Geometry check sheet. Reference: the model listing, model coordinates, mm. Face numbers are marked on the shaded views. A direction names the side the tool comes from. Coordinates: 2 decimals unless noted, no trailing zeros. Write each loop counter-clockwise with the first axis right and the second up, starting at its lowest first coordinate (ties: lowest second). Pieces come first, ordered by that corner, then holes. Notation, with made-up numbers: M 18,3.25 L 55,3.25 A13 ccw 55,23.25 Z; hole C -39.5,-13.75 d1. An arc over 180 degrees is marked long. Answer as a JSON object with one key per item and string values. Group by question number.
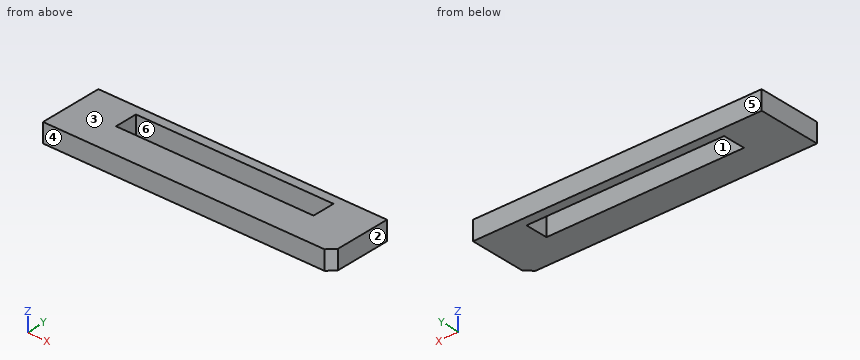
```python
from build123d import *

# Parameters (mm, degrees)
SKETCH_1_W          = 81.1
SKETCH_1_H          = 17.8
EXTRUDE_1_DEPTH     = 5.34
CHAMFER_1_SIZE      = 2
SKETCH_2_W          = 55.5
SKETCH_2_H          = 6.409449073
CUT_EXTRUDE_1_DEPTH = 6.34


with BuildPart() as part:
    # Эскиз1 → Бобышка-Вытянуть1 (new body)
    with BuildSketch(Plane.XY):
        with Locations((40.55, 8.9)):
            Rectangle(SKETCH_1_W, SKETCH_1_H)
    extrude(amount=EXTRUDE_1_DEPTH)

    # Фаска1
    chamfer_1_edges = [part.edges().sort_by_distance(p)[0] for p in [
        (81.1, 0, 2.67),
    ]]
    chamfer(chamfer_1_edges, length=CHAMFER_1_SIZE)

    # Эскиз2 → Вырез-Вытянуть1 (cut, through all)
    with BuildSketch(Plane.XY.offset(5.34)):
        with Locations((40.55, 12.038647742)):
            Rectangle(SKETCH_2_W, SKETCH_2_H)
    extrude(amount=-CUT_EXTRUDE_1_DEPTH, mode=Mode.SUBTRACT)


solid = part.part
```
1) Section check C-C (y = 12). Record the cut outline in (x, z), then the cut area to 3 significant figures.
2) Draft check along Y on the marked faces 3, 4, 5 and 6. Enter one of: +Y half, -Y half, draft (parallel to the pull), parting line (faces both ways), or undercut.
3) Section check A-A (x = 63). Record the cut outline in (y, z), then the cut area to 3 significant figures.
4) Set-up check for the marked faces 1 and 2: record each of +Z, -Z, +X, -X, +Y, -Y from which the full face is reachable in a straight line by a thin tool's end or side.
5) Section check B-B (z = 4). Record the cut outline in (x, y), then the cut area to 3 significant figures.
6) Go/stop test with a flat-tipped pin: pin 1 Ø1.5 at (y, z) = (16, 3.5) entering from -X. Record where the tip stops, or that it passes through.
7) Material ranges on probe 1 along X at (y, z) = (11.75, 4.65); probe 2 along Y at (x, z) = (44, 4.2); probe 3 along X at (y, z) = (1.5, 2.3), recorded low to high. Write a range as [from, to].
Entries:
{
 "1": {"outline": "M 0,0 L 12.8,0 L 12.8,5.34 L 0,5.34 Z; M 68.3,0 L 81.1,0 L 81.1,5.34 L 68.3,5.34 Z", "area": "137 mm^2"},
 "2": {"face 3": "draft", "face 4": "-Y half", "face 5": "+Y half", "face 6": "undercut"},
 "3": {"outline": "M 0,0 L 8.83,0 L 8.83,5.34 L 0,5.34 Z; M 15.24,0 L 17.8,0 L 17.8,5.34 L 15.24,5.34 Z", "area": "60.8 mm^2"},
 "4": {"face 1": "+Z, -Z", "face 2": "+Z, -Z, +X, +Y, -Y"},
 "5": {"outline": "M 0,0 L 79.1,0 L 81.1,2 L 81.1,17.8 L 0,17.8 Z; hole M 12.8,8.83 L 68.3,8.83 L 68.3,15.24 L 12.8,15.24 Z", "area": "1,090 mm^2"},
 "6": {"pin 1": "x = 0"},
 "7": {"probe 1": "[0, 12.8], [68.3, 81.1]", "probe 2": "[0, 8.83], [15.24, 17.8]", "probe 3": "[0, 80.6]"}
}
